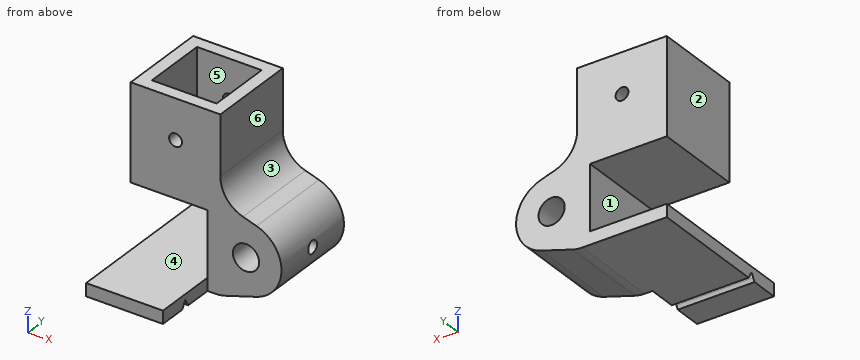
```python
from build123d import *

# Parameters (mm, degrees)
SKETCH1_R           = 4.1
BOSS_EXTRUDE1_DEPTH = 28
SKETCH2_W           = 20.2
SKETCH2_H           = 20.2
CUT_EXTRUDE1_DEPTH  = 25
SKETCH3_R           = 2
CUT_EXTRUDE2_DEPTH  = 78.071719846
FILLET1_R           = 10
SKETCH4_W           = 24
SKETCH4_H           = 4
BOSS_EXTRUDE2_DEPTH = 20
CUT_EXTRUDE3_DEPTH  = 66.556387942
CUT_EXTRUDE4_START  = 15.579105931
CUT_EXTRUDE4_DEPTH  = 7.520894069


# Read off the part's stored shape, not the designer's step: Cut-Extrude4
with BuildPart() as part:
    # Sketch1 → Boss-Extrude1 (new body)
    # profile 1 of 2: a face of its own
    with BuildSketch(Plane(origin=(0, 0, 0), x_dir=(1, 0, 0), z_dir=(0, 1, 0))):
        with BuildLine():
            Line((39.285734559, 50.702544431), (28, 54.2))
            Line((28, 54.2), (28, 26))
            Line((28, 26), (39.285734559, 29.497455569))
            ThreePointArc((39.285734559, 29.497455569), (47.1, 40.1), (39.285734559, 50.702544431))
        make_face()
        with Locations(Location((36, 40.1, 0), (0, 0, 270))):
            Circle(SKETCH1_R, mode=Mode.SUBTRACT)
    # profile 2 of 2: a face of its own
    with BuildSketch(Plane(origin=(0, 0, 0), x_dir=(1, 0, 0), z_dir=(0, 1, 0))):
        Polygon((28, 0), (28, 54.2), (0, 54.2), (0, 50.2), (24, 50.2), (24, 30), (0, 30), (0, 0), align=None)
    extrude(amount=BOSS_EXTRUDE1_DEPTH)

    # Sketch2 → Cut-Extrude1 (cut)
    with BuildSketch(Plane.XY):
        with Locations((14, 14)):
            Rectangle(SKETCH2_W, SKETCH2_H)
    extrude(amount=-CUT_EXTRUDE1_DEPTH, mode=Mode.SUBTRACT)

    # Sketch3 → Cut-Extrude2 (cut, through all)
    with BuildSketch(Plane(origin=(0, 28, 0), x_dir=(1, 0, 0), z_dir=(0, 1, 0))):
        with Locations(Location((14, 12.5, 0), (0, 0, 270))):
            Circle(SKETCH3_R)
    extrude(amount=-CUT_EXTRUDE2_DEPTH, mode=Mode.SUBTRACT)

    # Fillet1
    fillet1_edges = [part.edges().sort_by_distance(p)[0] for p in [
        (28, 14, -26),
        (28, 14, -54.2),
    ]]
    fillet(fillet1_edges, radius=FILLET1_R)

    # Sketch4 → Boss-Extrude2 (add)
    with BuildSketch(Plane.XZ):
        with Locations((12, -52.2)):
            Rectangle(SKETCH4_W, SKETCH4_H)
    extrude(amount=BOSS_EXTRUDE2_DEPTH)

    # Sketch5 → Cut-Extrude3 (cut, through all)
    with BuildSketch(Plane(origin=(24, 0, 0), x_dir=(0, 0, -1), z_dir=(1, 0, 0))):
        Polygon((54.2, -11.327905619), (54.2, -8.672094381), (53.2, -9.24944465), (53.2, -10.75055535), align=None)
        Polygon((53.2, -10.75055535), (53.2, -9.24944465), (51.9, -10), align=None)
    extrude(amount=-CUT_EXTRUDE3_DEPTH, mode=Mode.SUBTRACT)

    # Cut-Extrude4 outline → Cut-Extrude4 (cut)
    with BuildSketch(Plane(origin=(24, 0, 0), x_dir=(0, 0, -1), z_dir=(1, 0, 0)).offset(CUT_EXTRUDE4_START)):
        with BuildLine():
            add(Edge.make_bspline(
                [(38.1, 14), (38.1, 13.470320913), (38.317750981, 12.95373695), (39.054148284, 12.217509573), (39.57591962, 12.000304151), (40.621756395, 11.999696524), (41.14157679, 12.213335487), (41.886144514, 12.957531743), (42.099791904, 13.47657128), (42.100207779, 14.521837258), (41.883895964, 15.043849972), (41.147138028, 15.78196788), (40.629992878, 15.999596004), (39.573060585, 16.00040283), (39.055030391, 15.78291354), (38.318631187, 15.047600747), (38.1, 14.529679087), (38.1, 14)],
                knots=[0, 0, 0, 0, 0.125, 0.125, 0.25, 0.25, 0.375, 0.375, 0.5, 0.5, 0.625, 0.625, 0.75, 0.75, 0.875, 0.875, 1, 1, 1, 1], degree=3))
        make_face()
    extrude(amount=CUT_EXTRUDE4_DEPTH, mode=Mode.SUBTRACT)


solid = part.part
```
Work out the finished part from the listing and answer in its coordinate system (mm). Face numbers are marked on the shaded views. A direction names the side the tool comes from. Round coordinates to 2 decimals unless told otherwise and drop trailing zeros. Loops run counter-clockwise (first coordinate to the right, second up) from the corner with the lowest first, then second, coordinate; pieces in that order, holes last.
(1) Find the intervals of material crossed by L1, parallel to Y at x = 11.5, z = -23.5; L2, parallel to Z at x = 7, y = 22; L3, parallel to X at y = 2.9, z = -12.5, in increasing order.
Computed values:
L1: y = 0 to 3.9, 24.1 to 28
L2: z = -54.2 to -50.2, -30 to -25
L3: x = 0 to 12, 16 to 28
(2) The part is cut by section B-B, the plane y = 6.5. Give the vertices of the cut face in (x, z).
Computed values:
outline: (0, -54.2) - (26.49, -54.2) arc R10 ccw to (29.45, -53.75) - (39.29, -50.7) arc R11.1 ccw to (39.29, -29.5) - (35.04, -28.18) arc R10 cw to (28, -18.63) - (28, 0) - (24.1, 0) - (24.1, -25) - (3.9, -25) - (3.9, 0) - (0, 0) - (0, -30) - (24, -30) - (24, -50.2) - (0, -50.2) - close; hole circle Ø8.2 at (36, -40.1)
(3) Each of these flat-tipped pins is pushed along its axis until it touches: P1, Ø12, axis at x = 10.5, z = -33.5, coming from the -Y side; P2, Ø6, axis at x = 14, y = 12.5, coming from the +Z side; P3, Ø3, axis at y = -9.5, z = -52, coming from the +X side; P4, Ø3, axis at x = 8.5, z = -33, coming from the -Y side. Where does it stop, or does it pass through?
Computed values:
P1: stops at y = 0
P2: stops at z = -25
P3: stops at x = 24
P4: passes through
(4) The part is cut by section C-C, the plane x = 14. Give the vertices of the cut face in (y, z), and give its area (3 significant figures).
Computed values:
outline: (-20, -54.2) - (-11.33, -54.2) - (-10, -51.9) - (-8.67, -54.2) - (28, -54.2) - (28, -50.2) - (-20, -50.2) - close; (0, -30) - (28, -30) - (28, -14.5) - (24.1, -14.5) - (24.1, -25) - (3.9, -25) - (3.9, -14.5) - (0, -14.5) - close; (0, -10.5) - (3.9, -10.5) - (3.9, 0) - (0, 0) - close; (24.1, -10.5) - (28, -10.5) - (28, 0) - (24.1, 0) - close
area: 493 mm2
(5) The part is cut by section D-D, the plane z = -23. Give the vertices of the cut face in (x, y).
Computed values:
outline: (0, 0) - (29.01, 0) - (29.01, 28) - (0, 28) - close; hole (3.9, 3.9) - (24.1, 3.9) - (24.1, 24.1) - (3.9, 24.1) - close
(6) The mould has two halves that part along Z. Classify the marked faces 1, 2 and 3: pulls with the +Z half, pulls with the -Z half, needs draft (parallel to the pull), parting line crosses it, or undercut.
Computed values:
face 1: undercut
face 2: needs draft
face 3: pulls with the +Z half
(7) The part is cut by section A-A, the plane z = -12.5. Give the vertices of the cut face in (x, y), and give its area (3 significant figures).
Computed values:
outline: (0, 0) - (12, 0) - (12, 3.9) - (3.9, 3.9) - (3.9, 24.1) - (12, 24.1) - (12, 28) - (0, 28) - close; (16, 0) - (28, 0) - (28, 28) - (16, 28) - (16, 24.1) - (24.1, 24.1) - (24.1, 3.9) - (16, 3.9) - close
area: 345 mm2
(8) For the marked faces 4, 5 and 6, determine the directions among +Z, -Z, +X, -X, +Y, -Y from which every point of the face is accessible in a straight line to the end or side of a thin tool.
Computed values:
face 4: -X, +Y, -Y
face 5: +Z
face 6: +Z, +X, +Y, -Y
